Geometry check sheet. Reference: drawing and pictorial views, mm from the part's lowest x, y, z. Round coordinates to 2 decimals unless told otherwise and drop trailing zeros. Write each loop counter-clockwise with the first axis right and the second up, starting at its lowest first coordinate (ties: lowest second). Pieces come first, ordered by that corner, then holes. Notation, with made-up numbers: M -13,58 L 29,58 A22 ccw 29,65 Z; hole C 65,59.5 d11. An arc over 180 degrees is marked long. Put each result on its own line as item: value. Start each with the question number.
(1) Gauge pin test, flat ends, axial feed: pin 1 (1.1 mm diameter, centred on x = 3, y = 13.5, fed in from +Z); pin 2 (0.8 mm diameter, centred on x = 1, y = 9.5, fed in from +Z); pin 3 (1.5 mm diameter, centred on y = 8.5, z = 3, fed in from -X). Record the tip position at first contact, or that the pin passes through.
(2) Mould release check, pull along Y, two halves, no side actions. Record for the marked faces 1, 2, 3 and 4: pulls with the +Y half, pulls with the -Y half, needs draft (parallel to the pull), parting line crosses it, or undercut.
(3) Material ranges on probe 1 along Y at (x, z) = (2.5, 1.85); probe 2 along Z at (x, y) = (4, 4.75); probe 3 along X at (y, z) = (6.25, 3), recorded low to high.
(4) Section check A-A on x = 0.75. Record the cut outline in (y, z), then the cut area to 3 significant figures.
(5) Section check B-B on z = 1.85. Record the cut outline in (x, y), then the cut area to 3 significant figures.
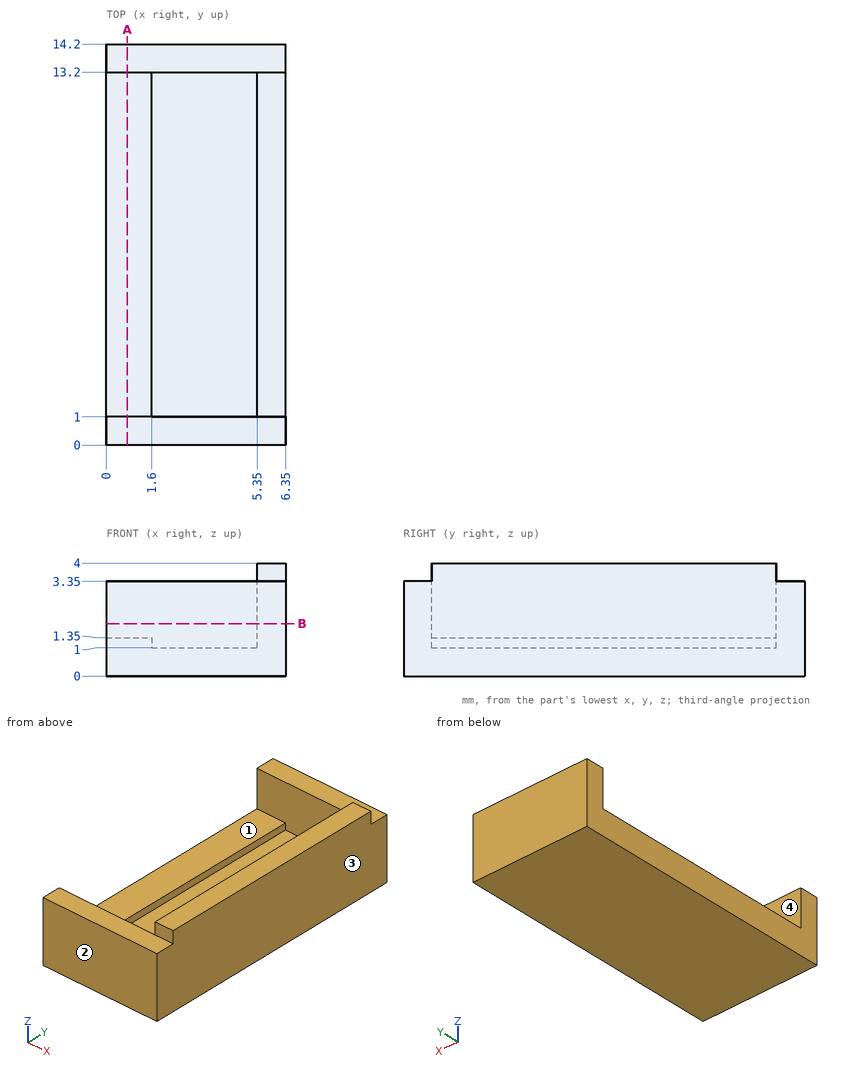
Answers follow:
1. pin 1: stops at z = 3.35
1. pin 2: stops at z = 1.35
1. pin 3: stops at x = 5.35
2. face 1: undercut
2. face 2: pulls with the -Y half
2. face 3: needs draft
2. face 4: undercut
3. probe 1: y = 0 to 1, 13.2 to 14.2
3. probe 2: z = 0 to 1
3. probe 3: x = 5.35 to 6.35
4. outline: M 0,0 L 14.2,0 L 14.2,3.35 L 13.2,3.35 L 13.2,1.35 L 1,1.35 L 1,3.35 L 0,3.35 Z
4. area: 23.2 mm^2
5. outline: M 0,0 L 6.35,0 L 6.35,14.2 L 0,14.2 L 0,13.2 L 5.35,13.2 L 5.35,1 L 0,1 Z
5. area: 24.9 mm^2
